CAD build for the part. Positions are in the model's coordinates, mm. A direction names the side the tool comes from. Coordinates: 2 decimals unless noted, no trailing zeros. Loops run counter-clockwise (first coordinate to the right, second up) from the corner with the lowest first, then second, coordinate; pieces in that order, holes last. Notation, with made-up numbers: (42, -39.5) -> (61, -39.5) arc R29 ccw to (61, -18.5) -> close; hole circle Ø9 at (82, 22). An arc over 180 degrees is marked (long way). Answer as a JSON object with one key per item and string values. Group by question number.
from build123d import *

# Parameters (mm, degrees)
STRUCTURAL_MEMBER1_DEPTH = 50
SKETCH16_R               = 2.5
CUT_EXTRUDE2_DEPTH       = 20
CUT_EXTRUDE7_REACH       = 116.8
CUT_EXTRUDE8_REACH       = 116.708
SKETCH23_R               = 2.1
CUT_EXTRUDE9_REACH       = 116.8
CUT_EXTRUDE10_REACH      = 112.716
SKETCH25_R               = 2.3
SKETCH26_R               = 6
CUT_EXTRUDE11_DEPTH      = 115.799827021


with BuildPart() as part:
    # Sketch14 → Structural Member1 (new body)
    with BuildSketch(Plane.YZ.offset(-25)):
        with BuildLine():
            Line((-11.999992417, -11.999998055), (72.000007583, -11.999998055))
            ThreePointArc((72.000007583, -11.999998055), (72.707114364, -11.707104836), (73.000007583, -10.999998055))
            Line((73.000007583, -10.999998055), (73.000007583, -3.999995305))
            ThreePointArc((73.000007583, -3.999995305), (72.707113392, -3.292890301), (72.000007583, -2.999998055))
            Line((72.000007583, -2.999998055), (23.000007583, -2.999998055))
            Line((23.000007583, -2.999998055), (-2.999992417, 23.000001945))
            Line((-2.999992417, 23.000001945), (-2.999992417, 72.000001945))
            ThreePointArc((-2.999992417, 72.000001945), (-3.292885636, 72.707108727), (-3.999992417, 73.000001945))
            Line((-3.999992417, 73.000001945), (-10.999992417, 73.000001945))
            ThreePointArc((-10.999992417, 73.000001945), (-11.707099198, 72.707108727), (-11.999992417, 72.000001945))
            Line((-11.999992417, 72.000001945), (-11.999992417, -11.999998055))
        make_face()
        with BuildLine():
            Line((0.999999969, -6.999999689), (17.221834624, -6.999999689))
            ThreePointArc((17.221834624, -6.999999689), (19.069593689, -5.765366553), (18.636048187, -3.585786126))
            Line((18.636048187, -3.585786126), (-3.585808896, 18.636070956))
            ThreePointArc((-3.585808896, 18.636070956), (-5.765389323, 19.069616459), (-7.000022459, 17.221857394))
            Line((-7.000022459, 17.221857394), (-7.000022459, 1.000002257))
            ThreePointArc((-7.000022459, 1.000002257), (-6.707129334, 0.29289557), (-6.000022726, 2.257e-06))
            Line((-6.000022726, 2.257e-06), (-4.974936959, 2.257e-06))
            ThreePointArc((-4.974936959, 2.257e-06), (-4.639527617, 0.129191559), (-4.477443471, 0.449999963))
            ThreePointArc((-4.477443471, 0.449999963), (-2.784112909, 3.535352218), (0.612237786, 4.458157119))
            ThreePointArc((0.612237786, 4.458157119), (0.960727975, 4.239434815), (1.027186757, 3.833395301))
            Line((1.027186757, 3.833395301), (0.660400741, 2.464528966))
            ThreePointArc((0.660400741, 2.464528966), (0.468097556, 2.187100615), (0.143315125, 2.095104001))
            ThreePointArc((0.143315125, 2.095104001), (-1.484932492, -1.484915989), (2.095105594, 0.14329184))
            ThreePointArc((2.095105594, 0.14329184), (2.18710419, 0.46807097), (2.464530895, 0.6603719))
            Line((2.464530895, 0.6603719), (3.83339913, 1.027158555))
            ThreePointArc((3.83339913, 1.027158555), (4.2394351, 0.960702167), (4.458159824, 0.612218085))
            ThreePointArc((4.458159824, 0.612218085), (3.535346067, -2.784120721), (0.449999963, -4.477443471))
            ThreePointArc((0.449999963, -4.477443471), (0.129190042, -4.639526994), (-3.1e-08, -4.974937189))
            Line((-3.1e-08, -4.974937189), (-3.1e-08, -5.999999623))
            ThreePointArc((-3.1e-08, -5.999999623), (0.292893164, -6.707106447), (0.999999969, -6.999999689))
        make_face(mode=Mode.SUBTRACT)
    extrude(amount=STRUCTURAL_MEMBER1_DEPTH)

    # Sketch16 → Cut-Extrude2 (cut)
    with BuildSketch(Plane(origin=(25, 0, 0), x_dir=(0, 0, -1), z_dir=(1, 0, 0))):
        with Locations((7.499998055, -7.499992417)):
            Circle(SKETCH16_R)
        with Locations((-39.744001945, -7.499992417)):
            Circle(SKETCH16_R)
        with Locations((7.499998055, 39.744007583)):
            Circle(SKETCH16_R)
    extrude(amount=-CUT_EXTRUDE2_DEPTH, mode=Mode.SUBTRACT)

    # Sketch18 → Cut-Revolve1 (revolve, cut)
    with BuildSketch(Plane(origin=(0, 2.977207172, 29.266802357), x_dir=(-1, 0, 0), z_dir=(0, 0.7071067811865477, 0.7071067811865475))):
        Polygon((-25, -38.589555017), (19, -38.589555017), (19, -21.764555017), (25, -21.764555017), (25, -18.589555017), (-25, -18.589555017), align=None)
    revolve(axis=Axis((25, 16.122007583, 16.122001945), (1, 0, 0)), mode=Mode.SUBTRACT)

    # Sketch22 → Cut-Extrude7 (cut, up to next)
    with BuildSketch(Plane(origin=(0, 0, -11.999998055), x_dir=(-1, 0, 0), z_dir=(0, 0, -1)), mode=Mode.PRIVATE) as cut_extrude7_sk1:
        with BuildLine():
            Line((11.825, 4.747007583), (-6.825, 4.747007583))
            ThreePointArc((-6.825, 4.747007583), (-9.07006403, 5.676943553), (-10, 7.922007583))
            Line((-10, 7.922007583), (-10, 30.922007583))
            ThreePointArc((-10, 30.922007583), (-9.07006403, 33.167071613), (-6.825, 34.097007583))
            Line((-6.825, 34.097007583), (11.825, 34.097007583))
            ThreePointArc((11.825, 34.097007583), (14.07006403, 33.167071613), (15, 30.922007583))
            Line((15, 30.922007583), (15, 7.922007583))
            ThreePointArc((15, 7.922007583), (14.07006403, 5.676943553), (11.825, 4.747007583))
        make_face()
    cut_extrude7_tool1 = extrude(cut_extrude7_sk1.sketch, amount=-CUT_EXTRUDE7_REACH, mode=Mode.PRIVATE) & part.part
    add(cut_extrude7_tool1.solids().sort_by_distance((-2.5, 19.422008, -11.999998))[0], mode=Mode.SUBTRACT)

    # Sketch23 → Cut-Extrude8 (cut, up to next)
    with BuildSketch(Plane.ZY.offset(25), mode=Mode.PRIVATE) as cut_extrude8_sk1:
        with Locations((-9.499998872, 11.922007583)):
            Circle(SKETCH23_R)
    cut_extrude8_tool1 = extrude(cut_extrude8_sk1.sketch, amount=-CUT_EXTRUDE8_REACH, mode=Mode.PRIVATE) & part.part
    # Sketch23 → Cut-Extrude8 (cut, up to next)
    with BuildSketch(Plane.ZY.offset(25), mode=Mode.PRIVATE) as cut_extrude8_sk2:
        with Locations((-7.499998055, 26.922007583)):
            Circle(SKETCH23_R)
    cut_extrude8_tool2 = extrude(cut_extrude8_sk2.sketch, amount=-CUT_EXTRUDE8_REACH, mode=Mode.PRIVATE) & part.part
    add(cut_extrude8_tool1.solids().sort_by_distance((-25, 11.922008, -9.499999))[0], mode=Mode.SUBTRACT)
    add(cut_extrude8_tool2.solids().sort_by_distance((-25, 26.922008, -7.499998))[0], mode=Mode.SUBTRACT)

    # Sketch24 → Cut-Extrude9 (cut, up to next)
    with BuildSketch(Plane.XZ.offset(11.999992417), mode=Mode.PRIVATE) as cut_extrude9_sk1:
        with BuildLine():
            Line((6.825, 8.000001945), (-11.825, 8.000001945))
            ThreePointArc((-11.825, 8.000001945), (-14.07006403, 8.929937915), (-15, 11.175001945))
            Line((-15, 11.175001945), (-15, 29.825001945))
            ThreePointArc((-15, 29.825001945), (-14.07006403, 32.070065976), (-11.825, 33.000001945))
            Line((-11.825, 33.000001945), (6.825, 33.000001945))
            ThreePointArc((6.825, 33.000001945), (9.07006403, 32.070065976), (10, 29.825001945))
            Line((10, 29.825001945), (10, 11.175001945))
            ThreePointArc((10, 11.175001945), (9.07006403, 8.929937915), (6.825, 8.000001945))
        make_face()
    cut_extrude9_tool1 = extrude(cut_extrude9_sk1.sketch, amount=-CUT_EXTRUDE9_REACH, mode=Mode.PRIVATE) & part.part
    # Sketch24 → Cut-Extrude9 (cut, up to next)
    with BuildSketch(Plane.XZ.offset(11.999992417), mode=Mode.PRIVATE) as cut_extrude9_sk2:
        with BuildLine():
            Line((25, 73.000001945), (-15, 73.000001945))
            Line((-15, 73.000001945), (-15, 48.325001945))
            ThreePointArc((-15, 48.325001945), (-14.07006403, 46.079937915), (-11.825, 45.150001945))
            Line((-11.825, 45.150001945), (25, 45.150001945))
            Line((25, 45.150001945), (25, 73.000001945))
        make_face()
    cut_extrude9_tool2 = extrude(cut_extrude9_sk2.sketch, amount=-CUT_EXTRUDE9_REACH, mode=Mode.PRIVATE) & part.part
    add(cut_extrude9_tool1.solids().sort_by_distance((-2.5, -11.999992, 20.500002))[0], mode=Mode.SUBTRACT)
    add(cut_extrude9_tool2.solids().sort_by_distance((5.037534, -11.999992, 59.100716))[0], mode=Mode.SUBTRACT)

    # Sketch25 → Cut-Extrude10 (cut, up to next)
    with BuildSketch(Plane(origin=(-15, 0, 0), x_dir=(0, 0, -1), z_dir=(1, 0, 0)), mode=Mode.PRIVATE) as cut_extrude10_sk1:
        with Locations((-67.000001945, -7.499992417)):
            Circle(SKETCH25_R)
    cut_extrude10_tool1 = extrude(cut_extrude10_sk1.sketch, amount=-CUT_EXTRUDE10_REACH, mode=Mode.PRIVATE) & part.part
    # Sketch25 → Cut-Extrude10 (cut, up to next)
    with BuildSketch(Plane(origin=(-15, 0, 0), x_dir=(0, 0, -1), z_dir=(1, 0, 0)), mode=Mode.PRIVATE) as cut_extrude10_sk2:
        with Locations((-25.825001945, -7.499992417)):
            Circle(SKETCH25_R)
    cut_extrude10_tool2 = extrude(cut_extrude10_sk2.sketch, amount=-CUT_EXTRUDE10_REACH, mode=Mode.PRIVATE) & part.part
    add(cut_extrude10_tool1.solids().sort_by_distance((-15, -7.499992, 67.000002))[0], mode=Mode.SUBTRACT)
    add(cut_extrude10_tool2.solids().sort_by_distance((-15, -7.499992, 25.825002))[0], mode=Mode.SUBTRACT)

    # Sketch26 → Cut-Extrude11 (cut, through all)
    with BuildSketch(Plane.XZ.offset(11.999992417)):
        with Locations((-9.455, 53.912001945)):
            Circle(SKETCH26_R)
    extrude(amount=-CUT_EXTRUDE11_DEPTH, mode=Mode.SUBTRACT)


solid = part.part
Item 1: Drill centre lines: L1, parallel to Z at x = 5.5, y = 54; L2, parallel to Z at x = -8, y = 4. Where is each one in solid material? Low to high.
Item 2: 3-axis set-ups, long thin cutter, end or side, ignore diameter. For faces 1 (the cylindrical face through (9.05, -7.56, 32.09)), 2 (the flat face through (6, -8, 45.15)), 3 (the flat face through (-22.04, 7.68, 7.37)), 4 (the flat face through (0, 48, -3)), 5 (the flat face through (-15, 22, -8)): which of +Z, -Z, +X, -X, +Y, -Y reach the whole face in a straight line?
Item 3: Band-saw the part on C-C, the plane z = 39.5. List the corners of the cut face in (x, y).
Item 4: Band-saw the part on A-A, the plane x = -3.5. Count the separate pieces of the cut face and the enclosed holes in it, and give its area (3 significant figures).
Item 5: Band-saw the part on B-B, the plane y = 21. List the corners of the cut face in (x, z), and give its area (3 significant figures).
Item 6: Pull direction Y, two halves, no side cores. Call faces 6 (the flat face through (10, 22, -8)), 7 (the flat face through (11, -12, 21)), 8 (the flat face through (-25, 11, 6)): +Y half, -Y half, draft (parallel to the pull), parting line (faces both ways), or undercut.
Item 7: Flat gauge pins, fed straight in: P1, Ø2, axis at x = -6, y = 53, coming from the +Z side; P2, Ø4, axis at y = -8.5, z = -8.5, coming from the +X side; P3, Ø10, axis at x = -15, y = 27, coming from the +Z side; P4, Ø4, axis at x = -2, y = -10.5, coming from the +Z side. Where does each tip first touch, or does it go through?
Reply:
{
 "1": {"L1": "-12 to -3", "L2": "-12 to -7, -2.06 to 0.21"},
 "2": {"face 1": "+Y, -Y", "face 2": "+Z, +X, +Y, -Y", "face 3": "+X, -X", "face 4": "+Z, +X, -X, +Y", "face 5": "+Z, -Z"},
 "3": {"outline": "(-25, -12) -> (25, -12) -> (25, -9.99) -> (5, -9.99) -> (5, -5.01) -> (25, -5.01) -> (25, -3) -> (-25, -3) -> close"},
 "4": {"separate pieces": "3", "enclosed holes": "0", "area": "691 mm²"},
 "5": {"outline": "(-25, -12) -> (-15, -12) -> (-15, -3.27) -> (-19, -3.27) -> (-19, -1) -> (-25, -1) -> close; (10, -12) -> (25, -12) -> (25, -3.27) -> (10, -3.27) -> close", "area": "232 mm²"},
 "6": {"face 6": "undercut", "face 7": "-Y half", "face 8": "draft"},
 "7": {"P1": "z = -3", "P2": "x = 25", "P3": "z = -2.75", "P4": "z = 45.15"}
}
